Source: three-view drawing plus pictorial views. Frame: mm from the lowest corner of the part. A direction names the side the tool comes from. Coordinates: 2 decimals unless noted, no trailing zeros. Order: outer loops, then holes, each group sorted by start corner. A loop starts at its lowest first (then second) coordinate and runs counter-clockwise, first axis right, second up. Notation, with made-up numbers: M -25.75,87 L 16.25,87 A35 ccw 16.25,119 Z; hole C 38.5,-11 d4. An arc over 180 degrees is marked long. Use CSV: the item, a comma, the result in double quotes. Start each with the question number.
Q1. Access query for the marked faces 1, 2 and 3. Directions: +Z, -Z, +X, -X, +Y, -Y. A direction counts if a zero-diameter tool reaches every point of the face in a straight line with its end or side. Return the directions, or none.
Q2. Ray query, probe 1 along X at (y, z) = (1.45, 6); probe 2 along X at (y, z) = (4.35, 10.5); probe 3 along X at (y, z) = (1.1, 51). Return the intervals inside material, ascending.
Q3. Section query C-C, the plane z = 59.5. Output: boundary loops of the cut face in (x, y), and give its area (3 significant figures).
Q4. Section query A-A, the plane x = 25.4. State how many separate pieces and enclosed holes the cut face has, and give its area (3 significant figures).
Q5. First-contact query: P1, Ø1.8, axis at x = 8.5, y = 3, coming from the -Z side; P2, Ø0.7, axis at x = 13.5, y = 2.5, coming from the +Z side (1 decimal); P3, Ø1, axis at y = 5, z = 46, coming from the -X side. Flat tips, straight axial feed; report the tip coordinate or a pass-through.
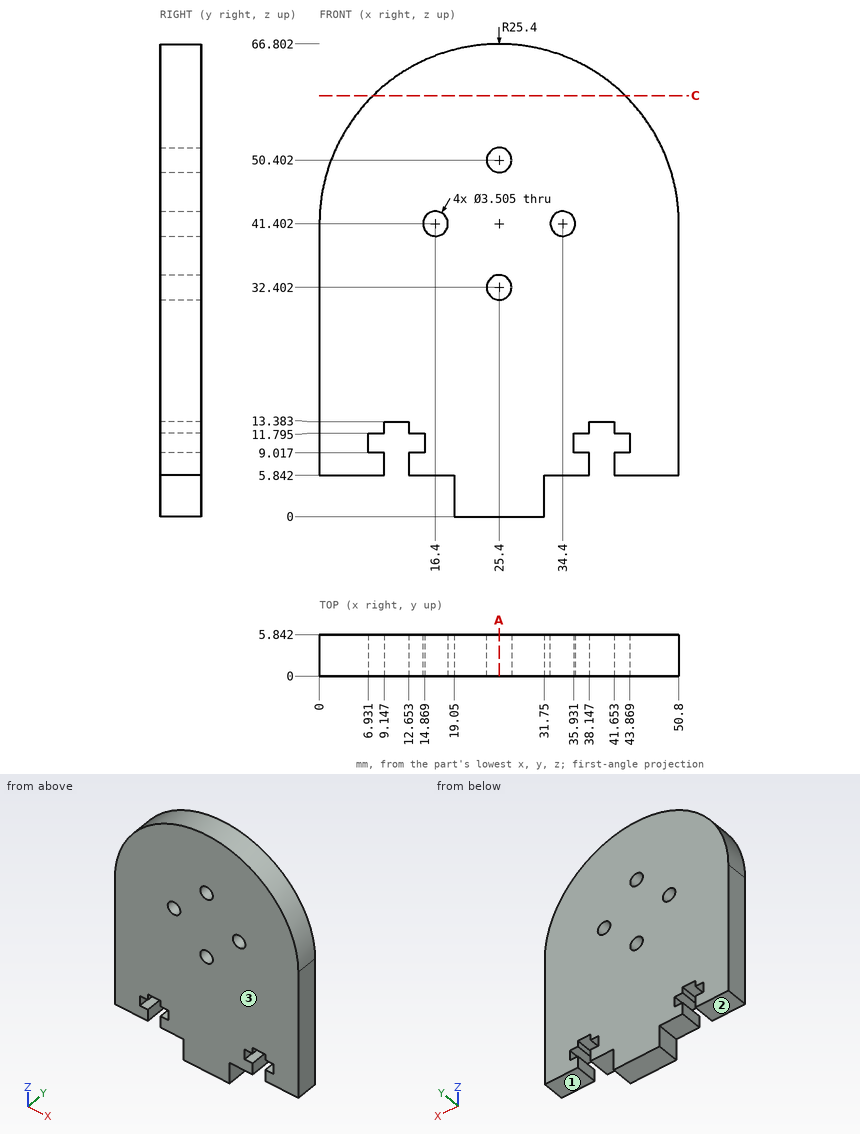
Responses:
1,face 1,"-Z, +X, +Y, -Y"
1,face 2,"-Z, -X, +Y, -Y"
1,face 3,"+Z, -Z, +X, -X, -Y"
2,probe 1,"x = 0 to 9.15, 12.65 to 38.15, 41.65 to 50.8"
2,probe 2,"x = 0 to 6.93, 14.87 to 35.93, 43.87 to 50.8"
2,probe 3,"x = 1.88 to 23.75, 27.05 to 48.92"
3,outline,"M 7.58,0 L 43.22,0 L 43.22,5.84 L 7.58,5.84 Z"
3,area,"208 mm²"
4,separate pieces,"3"
4,enclosed holes,"0"
4,area,"349 mm²"
5,P1,"stops at z = 5.84"
5,P2,"stops at z = 64"
5,P3,"stops at x = 0.33"
